Source: three-view drawing plus pictorial views. Frame: mm from the lowest corner of the part. Coordinates: 2 decimals unless noted, no trailing zeros. Loops run counter-clockwise (first coordinate to the right, second up) from the corner with the lowest first, then second, coordinate; pieces in that order, holes last. Notation, with made-up numbers: (34.25, 29.25) - (82.25, 29.25) arc R19 cw to (82.25, 57.25) - close; hole circle Ø3 at (-20, 50.5). An arc over 180 degrees is marked (long way). Return JSON: item names as keys, results as strings.
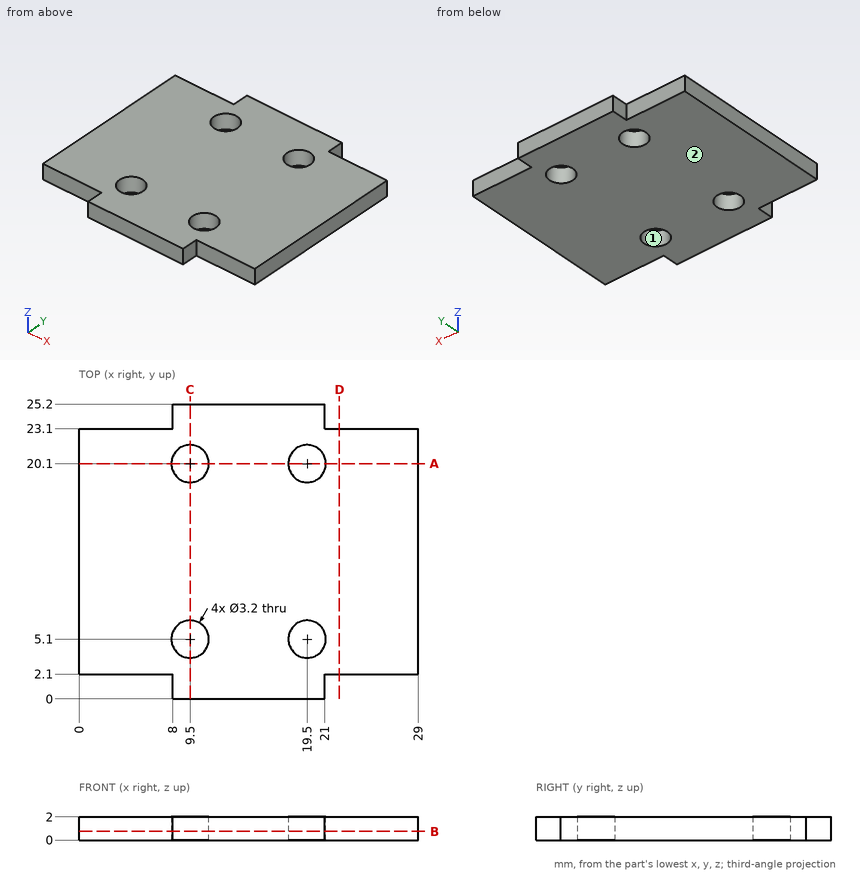
Item 1: Section query B-B, the plane z = 0.75. Return loops of the section in (x, y).
Worked out:
{"outline": "(0, 2.1) - (8, 2.1) - (8, 0) - (21, 0) - (21, 2.1) - (29, 2.1) - (29, 23.1) - (21, 23.1) - (21, 25.2) - (8, 25.2) - (8, 23.1) - (0, 23.1) - close; hole circle Ø3.2 at (9.5, 5.1); hole circle Ø3.2 at (9.5, 20.1); hole circle Ø3.2 at (19.5, 5.1); hole circle Ø3.2 at (19.5, 20.1)"}
Item 2: Section query A-A, the plane y = 20.1. Return loops of the section in (x, z), and give its area (3 significant figures).
Worked out:
{"outline": "(0, 0) - (7.9, 0) - (7.9, 2) - (0, 2) - close; (11.1, 0) - (17.9, 0) - (17.9, 2) - (11.1, 2) - close; (21.1, 0) - (29, 0) - (29, 2) - (21.1, 2) - close", "area": "45.2 mm^2"}
Item 3: Section query C-C, the plane x = 9.5. Return loops of the section in (y, z).
Worked out:
{"outline": "(0, 0) - (3.5, 0) - (3.5, 2) - (0, 2) - close; (6.7, 0) - (18.5, 0) - (18.5, 2) - (6.7, 2) - close; (21.7, 0) - (25.2, 0) - (25.2, 2) - (21.7, 2) - close"}
Item 4: Ray query, probe 1 along Y at (x, z) = (9.5, 1.25); probe 2 along X at (y, z) = (5.5, 1.1); probe 3 along Y at (x, z) = (18.75, 1.5). Return the intervals inside material, ascending. Write a range as from..to.
Worked out:
{"probe 1": "0..3.5, 6.7..18.5, 21.7..25.2", "probe 2": "0..7.95, 11.05..17.95, 21.05..29", "probe 3": "0..3.69, 6.51..18.69, 21.51..25.2"}
Item 5: First-contact query: pin 1 Ø1 at (y, z) = (1, 1) entering from +X; pin 2 Ø2.5 at (x, y) = (19.5, 20.1) entering from -Z; pin 3 Ø1 at (x, z) = (24, 1.5) entering from -Y; pin 4 Ø1 at (x, z) = (4.5, 0.5) entering from +Y. Flat tips, straight axial feed; report the tip coordinate or a pass-through.
Worked out:
{"pin 1": "x = 21", "pin 2": "through", "pin 3": "y = 2.1", "pin 4": "y = 23.1"}
Item 6: Mould query, pull axis X, two halves, no side actions, for the marked faces 1 and 2. Classes: +X half, -X half, draft (parallel to the pull), parting line (faces both ways), or undercut.
Worked out:
{"face 1": "undercut", "face 2": "draft"}
Item 7: Section query D-D, the plane x = 22.25. Return loops of the section in (y, z), and give its area (3 significant figures).
Worked out:
{"outline": "(2.1, 0) - (23.1, 0) - (23.1, 2) - (2.1, 2) - close", "area": "42.0 mm^2"}
